Could you check a few things on this model? Use its own coordinates, in mm. A direction names the side the tool comes from. Coordinates: 2 decimals unless noted, no trailing zeros. Write each loop counter-clockwise with the first axis right and the second up, starting at its lowest first coordinate (ties: lowest second). Pieces come first, ordered by that corner, then holes.
```python
from build123d import *

# Parameters (mm, degrees)
CHAMFER1_SIZE = 0.1


with BuildPart() as part:
    # Sketch1 → Revolve1 (revolve)
    with BuildSketch(Plane(origin=(0, 0, 0), x_dir=(0, 0, -1), z_dir=(1, 0, 0)), mode=Mode.PRIVATE) as revolve1_sk:
        with BuildLine():
            Line((-2, 2), (2, 2))
            Line((2, 2), (2, 2.6))
            Line((2, 2.6), (1.594951068, 2.6))
            ThreePointArc((1.594951068, 2.6), (2, 3.75), (1.594951068, 4.9))
            Line((1.594951068, 4.9), (2, 4.9))
            Line((2, 4.9), (2, 6.25))
            Line((2, 6.25), (1.04, 6.25))
            Line((1.04, 6.25), (1.04, 5.5))
            Line((1.04, 5.5), (-2, 5.5))
            Line((-2, 5.5), (-2, 4.9))
            Line((-2, 4.9), (-1.594951068, 4.9))
            ThreePointArc((-1.594951068, 4.9), (-2, 3.75), (-1.594951068, 2.6))
            Line((-1.594951068, 2.6), (-2, 2.6))
            Line((-2, 2.6), (-2, 2))
        make_face()
    revolve(revolve1_sk.sketch.rotate(Axis((0, 0, 0), (0, 0, -1)), 90), axis=Axis((0, 0, 0), (0, 0, -1)))

    # Chamfer1
    chamfer1_edges = [part.edges().sort_by_distance(p)[0] for p in [
        (-5.5, 0, 2),
        (-6.25, 0, -1.04),
        (-6.25, 0, -2),
    ]]
    chamfer(chamfer1_edges, length=CHAMFER1_SIZE)


solid = part.part
```
Item 1: I want a section at C-C, the plane z = 0.6. List the corners of the cut face in (x, y) for me.
Item 2: Which directions (+Z, -Z, +X, -X, +Y, -Y) give clear straight access to the entire face, cutting with the end or side of a thin tool? Please do faces 1 (the cylindrical face through (-1.19, 5.37, 0.45)), 2 (the flat face through (1, 5, 2)).
Item 3: If I drill on line 1 along Y through (x, z) = (0, 1.75); line 2 along Y through (x, z) = (0, 0.3); line 3 along Y through (x, z) = (0, -1.75), over which ranges is the centre line in solid material (lowest first)?
Item 4: Will this pin go through, and if not, where does the flat tip stop? pin 1 Ø1.5 at (y, z) = (-1, -0.5) entering from +X.
Item 5: If we mould it in two halves opening along Y, with no side actions, what happens to faces 3 (the flat face through (1, 2, 2)), 4 (the cylindrical face through (5.96, -1.88, -1.51)), 5 (the cylindrical face through (-3.612, -3.312, 1.795))? For each: released by +Y, released by -Y, zero draft, split by the parting line, or undercut.
Taken from the geometry:
1. outline: circle Ø11 at (0, 0); hole circle Ø4 at (0, 0)
2. face 1: +Z
2. face 2: +Z, +X, -X, +Y, -Y
3. line 1: y = -5.5 to -4.9, -4.67 to -2.83, -2.6 to -2, 2 to 2.6, 2.83 to 4.67, 4.9 to 5.5
3. line 2: y = -5.5 to -2, 2 to 5.5
3. line 3: y = -6.25 to -4.9, -4.67 to -2.83, -2.6 to -2, 2 to 2.6, 2.83 to 4.67, 4.9 to 6.25
4. pin 1: stops at x = 6.22
5. face 3: zero draft
5. face 4: split by the parting line
5. face 5: undercut
